from build123d import *

# Parameters (mm, degrees)
F0_W          = 80
F0_H          = 35
F1_DEPTH      = 15
F3_START      = 4
F2_W          = 80
F2_H          = 40
F3_DEPTH      = 21
F5_DEPTH      = 25
F5_DEPTH_BACK = 25
F6_R          = 2.5
F7_DEPTH      = 25
F7_DEPTH_BACK = 25


with BuildPart() as f1:
    # F0 (on Front) → F1 (new body)
    with BuildSketch(Plane.XZ):
        with Locations((-40, 17.5)):
            Rectangle(F0_W, F0_H)
    extrude(amount=F1_DEPTH)

    # F2 (on Front) → F3 (cut)
    with BuildSketch(Plane.XZ.offset(F3_START)):
        with Locations((-46, 9)):
            Rectangle(F2_W, F2_H)
    extrude(amount=F3_DEPTH, mode=Mode.SUBTRACT)

    # F4 (on Front) → F5 (cut, two sides)
    with BuildSketch(Plane.XZ) as f5_sk:
        with BuildLine():
            Line((-6.1243288219, -12.5113828104), (-6.1243288219, 0))
            ThreePointArc((-6.1243288219, 0), (-40.2652870135, 21.5150124091), (-79.961232841, 28.7767387927))
            Line((-79.961232841, 28.7767387927), (-95.1284343701, 28.6287205464))
            Line((-95.1284343701, 28.6287205464), (-94.7269439607, -12.5113828104))
            Line((-94.7269439607, -12.5113828104), (-6.1243288219, -12.5113828104))
        make_face()
    extrude(amount=F5_DEPTH, mode=Mode.SUBTRACT)
    extrude(f5_sk.sketch, amount=-F5_DEPTH_BACK, mode=Mode.SUBTRACT)

    # F6 (on Right) → F7 (cut, two sides)
    with BuildSketch(Plane.YZ) as f7_sk:
        with Locations((-9.5, 20)):
            Circle(F6_R)
        with BuildLine():
            ThreePointArc((-9.5, 7.5), (-7.732233047, 8.232233047), (-7, 10))
            ThreePointArc((-7, 10), (-11.267766953, 11.767766953), (-9.5, 7.5))
        make_face()
    extrude(amount=F7_DEPTH, mode=Mode.SUBTRACT)
    extrude(f7_sk.sketch, amount=-F7_DEPTH_BACK, mode=Mode.SUBTRACT)


solid = f1.part
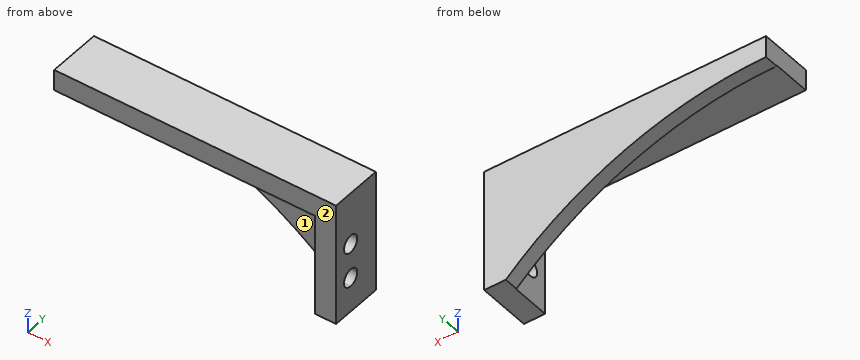
The model under review builds one solid part; all positions refer to its coordinate system, in mm. Face numbers are marked on the shaded views. A direction names the side the tool comes from. Round coordinates to 2 decimals unless told otherwise and drop trailing zeros. Write each loop counter-clockwise with the first axis right and the second up, starting at its lowest first coordinate (ties: lowest second). Pieces come first, ordered by that corner, then holes. Notation, with made-up numbers: M 33.5,7 L 89.5,7 A3 cw 89.5,12 Z; hole C 47.5,13 d2. An arc over 180 degrees is marked long. Answer as CSV lines item,"result". Start each with the question number.
Q1. Consider section A-A, the plane z = 19. Give the boundary of the cut face in (x, y), then the cut area to 3 significant figures.
Q2. Wall thickness on line 1 along Z through (x, y) = (-1.5, -9.5); line 2 along Y through (x, z) = (-3.8, 10); line 3 along Y through (x, z) = (-48.5, 27): over which ranges is each line inside the solid? List them lowest first.
Q3. Consider section B-B, the plane y = -14. Give the boundary of the cut face in (x, z), then the cut area to 3 significant figures.
Q4. Consider section C-C, the plane x = -51. Give the boundary of the cut face in (y, z), then the cut area to 3 significant figures.
Q5. Clearance check with flat-ended pins moving along their axes: P1, Ø8, axis at y = -9.5, z = 20, coming from the +X side; P2, Ø12, axis at x = -27, z = 20, coming from the -Y side; P3, Ø3.5, axis at x = -55.5, y = -9, coming from the -Z side; P4, Ø3, axis at y = -7, z = 24, coming from the -X side. State where each tip first meets the part, or that it passes through.
Q6. Tool access review of the marked faces 1 and 2: name each direction out of +Z, -Z, +X, -X, +Y, -Y from which nothing blocks a thin tool from reaching the whole face with its end or side.
Result set:
1,outline,"M -34.35,-4 L -6,-4 L -6,-7.21 L 0,-7.21 L 0,0 L -34.35,0 Z; M -6,-15 L 0,-15 L 0,-11.79 L -6,-11.79 Z"
1,area,"176 mm²"
2,line 1,"z = 0 to 7.5, 12.5 to 17.5, 22.5 to 35"
2,line 2,"y = -15 to -12, -7 to 0"
2,line 3,"y = -4 to 0"
3,outline,"M -80,29 L -6,29 L -6,0 L 0,0 L 0,35 L -80,35 Z"
3,area,"654 mm²"
4,outline,"M -15,29 L -4,29 L -4,25.05 L 0,25.05 L 0,35 L -15,35 Z"
4,area,"106 mm²"
5,P1,"stops at x = 0"
5,P2,"stops at y = -4"
5,P3,"stops at z = 29"
5,P4,"stops at x = -6"
6,face 1,"-Z, -X, -Y"
6,face 2,"+Z, -Z, +X, -X, -Y"
